The listing builds one solid part. Answer for the finished solid, in the listing's coordinates (mm). Face numbers are marked on the shaded views. A direction names the side the tool comes from. Coordinates: 2 decimals unless noted, no trailing zeros. Write each loop counter-clockwise with the first axis right and the second up, starting at its lowest first coordinate (ties: lowest second). Pieces come first, ordered by that corner, then holes.
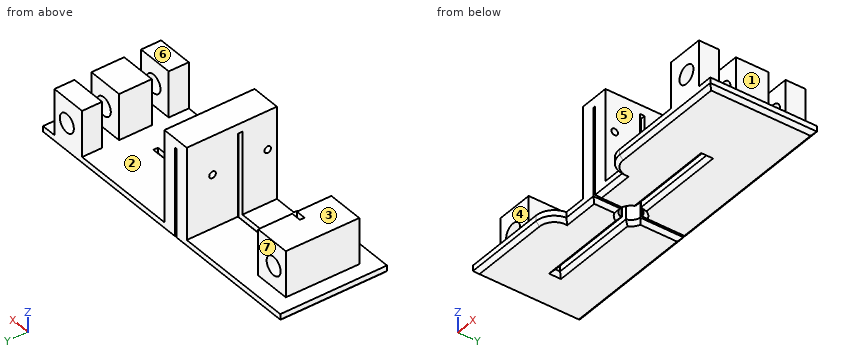
from build123d import *

# Parameters (mm, degrees)
SKETCH1_W           = 170
SKETCH1_H           = 58
BOSS_EXTRUDE1_DEPTH = 5
SKETCH2_W           = 28
SKETCH2_H           = 58
BOSS_EXTRUDE2_DEPTH = 25
CUT_EXTRUDE4_DEPTH  = 25
SKETCH6_W           = 16
SKETCH6_H           = 58
BOSS_EXTRUDE3_DEPTH = 50
SKETCH7_W           = 1.2
SKETCH7_H           = 58
CUT_EXTRUDE5_DEPTH  = 50
CUT_EXTRUDE6_DEPTH  = 50
SKETCH9_R           = 1.8
CUT_EXTRUDE7_DEPTH  = 20
HOLE3_START         = -20
HOLE3_OUTLINE_R     = 5
HOLE3_DEPTH         = 39.8
HOLE4_START         = -29
HOLE4_OUTLINE_R     = 5
HOLE4_DEPTH         = 58
SKETCH12_W          = 40
SKETCH12_H          = 9
CUT_EXTRUDE8_DEPTH  = 106.313816757
FILLET1_R           = 10
CHAMFER1_SIZE       = 2


# Read off the part's stored shape, not the designer's step: Hole3, Hole4
with BuildPart() as part:
    # Sketch1 → Boss-Extrude1 (new body)
    with BuildSketch(Plane.XY):
        Rectangle(SKETCH1_W, SKETCH1_H)
    extrude(amount=BOSS_EXTRUDE1_DEPTH)

    # Sketch2 → Boss-Extrude2 (add)
    with BuildSketch(Plane(origin=(0, 0, 5), x_dir=(-1, 0, 0), z_dir=(0, 0, -1))):
        with Locations((71, 0)):
            Rectangle(SKETCH2_W, SKETCH2_H)
        with Locations((-71, 0)):
            Rectangle(SKETCH2_W, SKETCH2_H)
    extrude(amount=-BOSS_EXTRUDE2_DEPTH)

    # Sketch3 → Cut-Extrude4 (cut)
    with BuildSketch(Plane.XY.offset(30)):
        Polygon((-57, -29), (-57, -20), (-77, -20), (-76.8, 19.8), (-57, 19.8), (-57, 29), (-85, 29), (-85, -29), align=None)
        Polygon((56, 8.9), (56, 18.1), (76.8, 18.1), (76.8, 29), (85, 29), (85, -29), (76.8, -29), (76.8, -18.1), (56, -18.1), (56, -8.9), (76.8, -8.9), (76.8, 8.9), align=None)
    extrude(amount=-CUT_EXTRUDE4_DEPTH, mode=Mode.SUBTRACT)

    # Sketch6 → Boss-Extrude3 (add)
    with BuildSketch(Plane.XY.offset(5)):
        with Locations((-10, 0)):
            Rectangle(SKETCH6_W, SKETCH6_H)
    extrude(amount=BOSS_EXTRUDE3_DEPTH)

    # Sketch7 → Cut-Extrude5 (cut)
    with BuildSketch(Plane(origin=(0, 0, 0), x_dir=(-1, 0, 0), z_dir=(0, 0, -1))):
        with Locations((10, 0)):
            Rectangle(SKETCH7_W, SKETCH7_H)
    extrude(amount=-CUT_EXTRUDE5_DEPTH, mode=Mode.SUBTRACT)

    # Sketch8 → Cut-Extrude6 (cut)
    with BuildSketch(Plane(origin=(0, 0, 0), x_dir=(-1, 0, 0), z_dir=(0, 0, -1))):
        with BuildLine():
            Line((15.356071321, 1.25), (62.5, 1.25))
            Line((62.5, 1.25), (62.5, -1.25))
            Line((62.5, -1.25), (15.356071321, -1.25))
            ThreePointArc((15.356071321, -1.25), (10, -5.5), (4.643928679, -1.25))
            Line((4.643928679, -1.25), (-42.5, -1.25))
            Line((-42.5, -1.25), (-42.5, 1.25))
            Line((-42.5, 1.25), (4.643928679, 1.25))
            ThreePointArc((4.643928679, 1.25), (10, 5.5), (15.356071321, 1.25))
        make_face()
    extrude(amount=-CUT_EXTRUDE6_DEPTH, mode=Mode.SUBTRACT)

    # Sketch9 → Cut-Extrude7 (cut)
    with BuildSketch(Plane.ZY.offset(18)):
        with Locations((34, 15)):
            Circle(SKETCH9_R)
        with Locations((34, -15)):
            Circle(SKETCH9_R)
    extrude(amount=-CUT_EXTRUDE7_DEPTH, mode=Mode.SUBTRACT)

    # Hole3 outline → Hole3 (cut)
    with BuildSketch(Plane(origin=(0, 0, 0), x_dir=(1, 0, 0), z_dir=(0, 1, 0)).offset(HOLE3_START)):
        with Locations((-68.081865543, -16.770132162)):
            Circle(HOLE3_OUTLINE_R)
    extrude(amount=HOLE3_DEPTH, mode=Mode.SUBTRACT)

    # Hole4 outline → Hole4 (cut)
    with BuildSketch(Plane(origin=(0, 0, 0), x_dir=(1, 0, 0), z_dir=(0, 1, 0)).offset(HOLE4_START)):
        with Locations((67.918134457, -16.770132162)):
            Circle(HOLE4_OUTLINE_R)
    extrude(amount=HOLE4_DEPTH, mode=Mode.SUBTRACT)

    # Sketch12 → Cut-Extrude8 (cut, through all)
    with BuildSketch(Plane(origin=(0, 0, 0), x_dir=(-1, 0, 0), z_dir=(0, 0, -1))):
        with Locations((10, -24.5)):
            Rectangle(SKETCH12_W, SKETCH12_H)
    extrude(amount=-CUT_EXTRUDE8_DEPTH, mode=Mode.SUBTRACT)

    # Fillet1
    # the kernel refuses this fillet: 10 mm, written as the material it takes off along each edge
    with BuildSketch(Plane(origin=(-30, -29, -24.874685928), x_dir=(0, 1, 0), z_dir=(0, 0, 1))) as fillet1_piece_1:
        with BuildLine():
            CenterArc((10, 9.949874371), FILLET1_R, 180, 84.260829523)
            Line((0, 9.949874371), (-0.2, 9.949874371))
            Line((-0.2, 9.949874371), (-0.2, 0))
            Line((-0.2, 0), (0, -0.2))
            ThreePointArc((0, -0.2), (4.5, -0.2), (8.98, -0.198997487))
            Line((8.98, -0.198997487), (9, 0))
        make_face()
    extrude(amount=54.749371855, mode=Mode.SUBTRACT)
    with BuildSketch(Plane(origin=(10, -29, -24.874685928), x_dir=(0, 1, 0), z_dir=(0, 0, 1))) as fillet1_piece_2:
        with BuildLine():
            CenterArc((10, -9.949874371), FILLET1_R, 95.739170477, 84.260829523)
            Line((0, -9.949874371), (-0.2, -9.949874371))
            Line((-0.2, -9.949874371), (-0.2, 0))
            Line((-0.2, 0), (0, 0.2))
            ThreePointArc((0, 0.2), (4.5, 0.2), (8.98, 0.198997487))
            Line((8.98, 0.198997487), (9, 0))
        make_face()
    extrude(amount=54.749371855, mode=Mode.SUBTRACT)

    # Chamfer1
    chamfer1_edges = [part.edges().sort_by_distance(p)[0] for p in [
        (-47.8, 29, 0),
        (-9.4, 17.233587387, 0),
        (-10.6, 17.233587387, 0),
        (-9.4, -12.733587387, 0),
        (-6.351049855, -4.115235453, 0),
        (-6.351049855, 4.115235453, 0),
        (18.928035661, 1.25, 0),
        (42.5, 0, 0),
        (18.928035661, -1.25, 0),
        (-13.648950145, 4.115235453, 0),
        (-13.648950145, -4.115235453, 0),
        (-38.928035661, -1.25, 0),
        (-62.5, 0, 0),
        (-38.928035661, 1.25, 0),
        (-10.6, -12.733587387, 0),
        (0.3, -20, 0),
        (-20.3, -20, 0),
        (-33.241670439, -26.416198487, 0),
        (52.474937186, -29, 0),
        (13.241670439, -26.416198487, 0),
        (37.8, 29, 0),
        (85, 0, 0),
        (-62.474937186, -29, 0),
        (-85, 0, 0),
    ]]
    chamfer(chamfer1_edges, length=CHAMFER1_SIZE)


solid = part.part
1. Flat-ended cylindrical pins translate along their axes: P1, Ø3, axis at y = 13.5, z = 36, coming from the +X side; P2, Ø4.5, axis at y = -12, z = 21.5, coming from the -X side; P3, Ø10, axis at x = -68.5, y = -4.5, coming from the +Z side. Find the tip coordinate at first contact, or state that the pin passes through.
Results found:
P1: stops at x = -2
P2: stops at x = -76.97
P3: stops at z = 30
2. For a pull along X with two mould halves and no side action, classify the marked faces 1, 2 and 3 as pulls with the +X half, pulls with the -X half, needs draft (parallel to the pull), parting line crosses it, or undercut.
Results found:
face 1: pulls with the +X half
face 2: undercut
face 3: needs draft
3. A tool of negligible diameter and unlimited length cuts with its end or side. For the marked faces 4, 5, 6 and 7, from which of +Z, -Z, +X, -X, +Y, -Y can it reach the whole face along a straight path? Write none if from no direction.
Results found:
face 4: +Z, -X, -Y
face 5: +Z, +Y, -Y
face 6: +Z, +X, +Y, -Y
face 7: +Z, -X, +Y
4. Find the intervals of material crossed by L1, parallel to Y at x = -15.75, z = 34; L2, parallel to Y at x = 67.5, z = 9; L3, parallel to X at y = 15, z = 41.5, in increasing order.
Results found:
L1: y = -20 to -16.8, -13.2 to -1.25, 1.25 to 13.2, 16.8 to 29
L2: y = -29 to -18.1, -8.9 to 8.9, 18.1 to 29
L3: x = -18 to -10.6, -9.4 to -2
5. Section B-B on y = -15 is taken. State how many separate pieces and enclosed holes the cut face has, then the cut area to 3 significant figures.
Results found:
separate pieces: 3
enclosed holes: 1
area: 1,950 mm2
6. Section A-A on z = 47 is taken. Give the vertices of the cut face in (x, y), then the cut area to 3 significant figures.
Results found:
outline: (-18, -20) - (-10.6, -20) - (-10.6, -5.47) arc R5.5 cw to (-15.36, -1.25) - (-18, -1.25) - close; (-18, 1.25) - (-15.36, 1.25) arc R5.5 cw to (-10.6, 5.47) - (-10.6, 29) - (-18, 29) - close; (-9.4, -20) - (-2, -20) - (-2, -1.25) - (-4.64, -1.25) arc R5.5 cw to (-9.4, -5.47) - close; (-9.4, 5.47) arc R5.5 cw to (-4.64, 1.25) - (-2, 1.25) - (-2, 29) - (-9.4, 29) - close
area: 631 mm2
